Design review of the part built by this model. Coordinates are the model's own, in mm. Face numbers are marked on the shaded views. A direction names the side the tool comes from. Give positions to 0.01 mm unless a question says otherwise; leave off trailing zeros. Order: outer loops, then holes, each group sorted by start corner. A loop starts at its lowest first (then second) coordinate and runs counter-clockwise, first axis right, second up. Notation, with made-up numbers: M -35.75,37 L -25.75,37 A33 ccw -25.75,74 Z; hole C 38,-12.75 d6. An arc over 180 degrees is marked long. Put each result on its own line as item: value. Start each with the question number.
from build123d import *

# Parameters (mm, degrees)
F1_DEPTH    = 10
F2_W        = 4.5836600475
F2_H        = 4
F3_DEPTH    = 25
F4_W        = 2.6
F4_H        = 5
F5_DEPTH    = 25
F6_R        = 3
F7_R        = 3
F8_R        = 1
F9_T1_DEPTH = 15
F9_T4_ANGLE = 90
F9_T6_ANGLE = 90


# Not quite as in the source:
# - a fillet or chamfer that OpenCascade refuses, or shapes differently, is made with other operations: its cross-section is extruded or revolved along the edge and cut away or added


with BuildPart() as f1:
    # F0 (on Top) → F1 (new body)
    with BuildSketch(Plane.XY):
        Polygon((4.5, 4), (0, 4), (-4.5, 4), (-4.5, 1), (-3, 1), (-3, 0), (-4.5, 0), (-10, 0), (-10, -20), (0, -20), (10, -20), (10, 0), (4.5, 0), (3, 0), (3, 1), (4.5, 1), align=None)
    extrude(amount=F1_DEPTH)

    # F2 (on face) → F3 (cut)
    with BuildSketch(Plane(origin=(-10, 0, 0), x_dir=(0, -1, 0), z_dir=(-1, 0, 0))):
        with Locations((-2.2918300238, 8)):
            Rectangle(F2_W, F2_H)
    extrude(amount=-F3_DEPTH, mode=Mode.SUBTRACT)

    # F4 (on face) → F5 (cut)
    with BuildSketch(Plane.YZ.offset(10)):
        with Locations((-17.3, 7.5)):
            Rectangle(F4_W, F4_H)
    extrude(amount=-F5_DEPTH, mode=Mode.SUBTRACT)

    # F6
    f6_edges = [f1.edges().sort_by_distance(p)[0] for p in [
        (3, 0.5, 0),
        (-3, 0.5, 6),
    ]]
    fillet(f6_edges, radius=F6_R)

    # F7
    f7_edges = [f1.edges().sort_by_distance(p)[0] for p in [
        (4.5, 2.5, 0),
        (-4.5, 2.5, 6),
    ]]
    fillet(f7_edges, radius=F7_R)

    # F8
    f8_edges = [f1.edges().sort_by_distance(p)[0] for p in [
        (-10, -8, 10),
        (10, -8, 10),
        (-10, -10, 0),
        (0, -20, 0),
        (10, -10, 0),
        (0, -18.6, 10),
        (0, -16, 10),
    ]]
    fillet(f8_edges, radius=F8_R)

    # F9: fillet of radius 2 on 2 edges, made by hand

    # F9_s2 → F9_t1 (cut)
    with BuildSketch(Plane.XY):
        with BuildLine():
            ThreePointArc((10, -18), (9.4142135624, -19.4142135624), (8, -20))
            Line((8, -20), (10, -20))
            Line((10, -20), (10, -18))
        make_face()
        with BuildLine():
            ThreePointArc((-10, -18), (-9.4142135624, -19.4142135624), (-8, -20))
            Line((-8, -20), (-10, -20))
            Line((-10, -20), (-10, -18))
        make_face()
    extrude(amount=F9_T1_DEPTH, mode=Mode.SUBTRACT)

    # F9_s3 → F9_t4 (revolve, cut)
    with BuildSketch(Plane.YZ.offset(-8)):
        with BuildLine():
            ThreePointArc((-19, 0), (-19.7071067812, 0.2928932188), (-20, 1))
            Line((-20, 1), (-20, 0))
            Line((-20, 0), (-19, 0))
        make_face()
    revolve(axis=Axis((-8, -18, 0), (0, 0, -1)), revolution_arc=F9_T4_ANGLE, mode=Mode.SUBTRACT)

    # F9_s5 → F9_t6 (revolve, cut)
    with BuildSketch(Plane.XZ.offset(18)):
        with BuildLine():
            ThreePointArc((9, 0), (9.7071067812, 0.2928932188), (10, 1))
            Line((10, 1), (10, 0))
            Line((10, 0), (9, 0))
        make_face()
    revolve(axis=Axis((8, -18, 0), (0, 0, -1)), revolution_arc=F9_T6_ANGLE, mode=Mode.SUBTRACT)


solid = f1.part
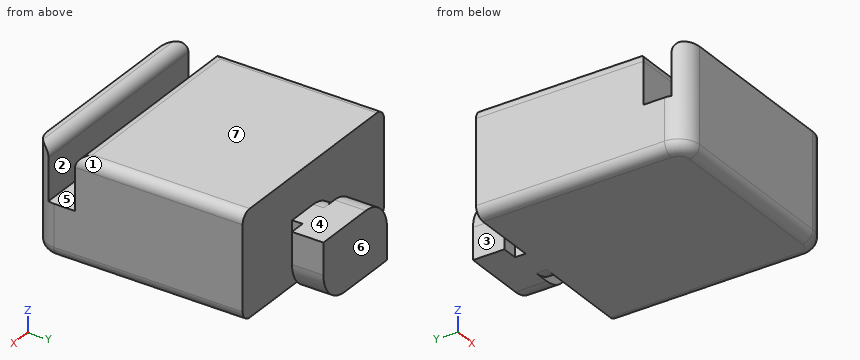
1. Insertion check: pin 1 (4.5 mm diameter, centred on x = 1.5, y = 2, fed in from +Z); pin 2 (0.9 mm diameter, centred on y = 2, z = 2, fed in from -X); pin 3 (0.8 mm diameter, centred on x = -4.5, y = -17.5, fed in from +Z); pin 4 (1.5 mm diameter, centred on y = 2, z = 5, fed in from +X). Each pin has a flat end and moves straight along its axis. Give the tip position at first contact, or say it passes through.
2. To check wall thickness, follow probe 1 along Y at (x, z) = (1, 5.5); probe 2 along Y at (x, z) = (-5.75, 7.75); probe 3 along Y at (x, z) = (5.75, 3.5). State the ranges of each line that lie inside material, in increasing order.
3. The part is to be moulded in two halves that separate along Y. For the marked faces 5, 6 and 7, say which applies: +Y half, -Y half, draft (parallel to the pull), parting line (faces both ways), or undercut.
4. Consider section A-A on z = 7. Give the boundary of the cut face in (x, y), then the cut area to 3 significant figures.
5. Machinability: for the marked faces 1, 2, 3 and 4, which of the approach directions +Z, -Z, +X, -X, +Y, -Y give a long, thin tool a straight path to every point of the face, cutting with its end or side? Answer none if there is none.
6. Consider section B-B on x = 7. Give the boundary of the cut face in (y, z).
7. Consider section C-C on y = -15.5. Give the boundary of the cut face in (x, z), then the cut area to 3 significant figures.
8. Consider section D-D on z = 2.5. Give the boundary of the cut face in (x, y).
Returned:
1. pin 1: stops at z = 10
1. pin 2: stops at x = -4.5
1. pin 3: stops at z = 5
1. pin 4: stops at x = 4.5
2. probe 1: y = -20 to -18.6, -16 to 4
2. probe 2: y = -20 to -18.6, -16 to 0
2. probe 3: y = -20 to 0
3. face 5: undercut
3. face 6: +Y half
3. face 7: draft
4. outline: M -10,-16 L 10,-16 L 10,0 L -10,0 Z; M -9.91,-18.6 A2 ccw -8,-20 L 8,-20 A2 ccw 9.91,-18.6 Z
4. area: 346 mm2
5. face 1: +Z, +X, +Y
5. face 2: +Z, +X, -X
5. face 3: +Z, -Z, -X, +Y
5. face 4: +Z, +X, -X, +Y
6. outline: M -20,1 A1 ccw -19,0 L 0,0 L 0,10 L -15,10 A1 ccw -16,9 L -16,5 L -18.6,5 L -18.6,9 A1 ccw -19.6,10 L -20,10 Z
7. outline: M -10,1 A1 ccw -9,0 L 9,0 A1 ccw 10,1 L 10,9 A1 ccw 9.5,9.87 L -9.5,9.87 A1 ccw -10,9 Z
7. area: 197 mm2
8. outline: M -10,-18 A2 ccw -8,-20 L 8,-20 A2 ccw 10,-18 L 10,0 L 2.96,0 L 2.96,1 L 4.46,1 L 4.46,4 L -4.5,4 L -4.5,1 L -3,1 L -3,0 L -10,0 Z
